Source: CAD feature listing. Evaluate the final solid. Frame: model axes, mm. Face numbers are marked on the shaded views. Round coordinates to 2 decimals unless told otherwise and drop trailing zeros. Order: outer loops, then holes, each group sorted by start corner. A loop starts at its lowest first (then second) coordinate and runs counter-clockwise, first axis right, second up. Notation, with made-up numbers: (76, 34) - (129, 34) arc R15 ccw to (129, 62) - close; hole circle Ø1 at (38, 22). An arc over 180 degrees is marked (long way). Use one line per item in the form item = value. Start each with the question number.
Q1. Cut plane B-B, the plane z = 13. Return the cut outline in (x, y), and give its area (3 significant figures).
Q2. Ray query, line 1 (Y direction, x = -58.5, z = 48); line 2 (Y direction, x = 20.5, z = 18). Return the intervals inside material, ascending. Write a range as [from, to].
Q3. Cut plane C-C, the plane y = 60.5. Return the cut outline in (x, z), and give its area (3 significant figures).
Q4. Draft query along Z for the marked faces 1, 2 and 3. Return one class per face: released by +Z, released by -Z, zero draft, split by the parting line, or undercut.
Q5. Pin query (flat end, axial travel): pin 1 Ø12 at (x, y) = (58.5, 54.5) entering from +Z; pin 2 Ø10 at (x, z) = (70.5, 53) entering from +Y; pin 3 Ø1.2 at (x, y) = (-38.5, 2.5) entering from -Z. Return the tip coordinate at first contact, or that it passes through.
from build123d import *

# Parameters (mm, degrees)
EXTRUDE_1_DEPTH      = 96
EXTRUDE_1_DEPTH_BACK = 96
SKETCH_1_W           = 1.5
SKETCH_1_H           = 8.5
FILLET_1_R           = 1.5


with BuildPart() as part:
    # 草圖1 → 擠出1 (new, two sides: drawn at the far end of the back side and taken through both)
    with BuildSketch(Plane.YZ.offset(-EXTRUDE_1_DEPTH_BACK)):
        Polygon((1.5, 17), (1.5, 17.621320344), (0, 17), align=None)
        Polygon((17.621320344, 1.5), (17, 1.5), (17, 0), align=None)
        with Locations((2.25, 106.75)):
            Rectangle(SKETCH_1_W, SKETCH_1_H)
        with Locations((110.35, 15.25)):
            Rectangle(SKETCH_1_W, SKETCH_1_H)
        Polygon((111.1, 11), (111.1, 1.5), (112.6, 1.5), (112.6, 19.5), (111.1, 19.5), align=None)
        Polygon((17.621320344, 1.5), (17, 1.5), (17, 0), (0, 17), (1.5, 17), (1.5, 17.621320344), align=None)
        Polygon((0, 111), (0, 17), (1.5, 17.621320344), (1.5, 102.5), (1.5, 111), align=None)
        Polygon((17.621320344, 1.5), (17, 0), (112.6, 0), (112.6, 1.5), (111.1, 1.5), align=None)
    extrude(amount=EXTRUDE_1_DEPTH + EXTRUDE_1_DEPTH_BACK)

    # 圓角1
    fillet_1_edges = [part.edges().sort_by_distance(p)[0] for p in [
        (0, 0, 111),
        (0, 3, 111),
        (0, 1.5, 17.621320344),
        (0, 17, 0),
        (0, 0, 17),
        (0, 17.621320344, 1.5),
        (0, 111.1, 1.5),
        (0, 112.6, 0),
        (0, 109.6, 19.5),
        (0, 112.6, 19.5),
    ]]
    fillet(fillet_1_edges, radius=FILLET_1_R - 0.0001)  # a hair under: the kernel refuses the full size


solid = part.part
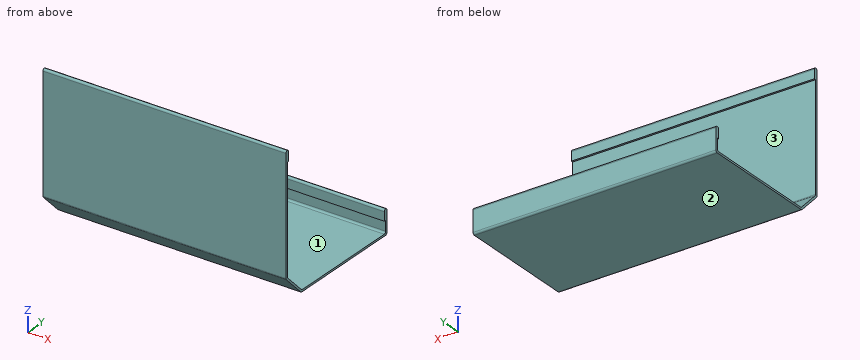
Completed:
q1.outline = (-96, 4) - (96, 4) - (96, 6.12) - (-96, 6.12) - close; (-96, 109.6) - (96, 109.6) - (96, 112.6) - (-96, 112.6) - close
q1.area = 983 mm2
q2.line_1 = [0, 1.5]
q2.line_2 = [0, 1.52], [109.6, 112.6]
q3.outline = (-96, 0) - (96, 0) - (96, 1.5) - (-96, 1.5) - close
q3.area = 288 mm2
q4.face_1 = released by +Z
q4.face_2 = released by -Z
q4.face_3 = undercut
q5.pin_1 = 1.5
q5.pin_2 = 1.5
q5.pin_3 = 13.9
